Could you check a few things on this model? Use its own coordinates, in mm. A direction names the side the tool comes from. Coordinates: 2 decimals unless noted, no trailing zeros. Write each loop counter-clockwise with the first axis right and the second up, starting at its lowest first coordinate (ties: lowest second). Pieces come first, ordered by that corner, then holes. Notation, with made-up numbers: M 67.5,2 L 114.5,2 A10 ccw 114.5,6 Z; hole C 40.5,1 d8. An arc over 180 degrees is marked long. Answer as CSV lines item,"result". Start each with the question number.
Item 1: Suppose I cut it at A-A, the plane x = 7. Write out the boundary of the cut face in (y, z), and give its area (3 significant figures).
Item 2: We'd pull the mould along Z, two halves only. Please class faces 1 (the flat face through (0, 16, 0)), 2 (the cylindrical face through (2.854, -0.056, 42.939)), 3 (the cylindrical face through (11.19, -0.06, 62.72)), 4 (the flat face through (7, 4, 44)): +Z half, -Z half, draft (parallel to the pull), parting line (faces both ways), or undercut.
Item 3: I'm going to push flat-ended pins straight in: P1, Ø9.5, axis at x = -6, y = 43.5, coming from the +Z side; P2, Ø2.5, axis at x = 0.5, y = 0, coming from the -Z side; P3, Ø1.3, axis at x = 6.5, y = -12.5, coming from the +Z side. Where does each tip first touch, or does it pass through?
Item 4: Suppose I cut it at B-B, the plane y = 1. Write out the boundary of the cut face in (x, z), and give its area (3 significant figures).
Item 5: Suppose I cut it at D-D, the plane z = 4. Write out the boundary of the cut face in (x, y).
Item 6: Suppose I cut it at C-C, the plane y = -19. Write out the boundary of the cut face in (x, z), and give its area (3 significant figures).
Item 7: If I drill on line 1 along Z through (x, y) = (9, -13); line 2 along X through (y, z) = (-3, 7); line 3 along X through (y, z) = (-2.5, 52), over which ranges is the centre line in solid material (lowest first)? Write a range as [from, to].
Item 8: On a 3-axis mill with a long thin cutter (end or side, diameter ignored), from which of +Z, -Z, +X, -X, +Y, -Y can I reach the whole of each face in a straight line? I mean faces 5 (the flat face through (10.5, 39, 28)), 6 (the flat face through (-8, -12, 31.4)), 7 (the flat face through (13, 43, 22)). Say none if no direction works.
```python
from build123d import *

# Parameters (mm, degrees)
SKETCH4_W            = 31.4
SKETCH4_H            = 31.4
SKETCH4_W_2          = 25.4
SKETCH4_H_2          = 25.4
BOSS_EXTRUDE3_DEPTH  = 30
SKETCH5_W            = 31.4
SKETCH5_H            = 31.4
BOSS_EXTRUDE4_DEPTH  = 5
SKETCH6_W            = 31.4
SKETCH6_H            = 8
BOSS_EXTRUDE5_DEPTH  = 5
BOSS_EXTRUDE6_DEPTH  = 8
SKETCH8_R            = 9.5
BOSS_EXTRUDE7_DEPTH  = 8
SKETCH9_W            = 31.4
SKETCH9_H            = 10
BOSS_EXTRUDE8_DEPTH  = 5
SKETCH10_W           = 31.4
SKETCH10_H           = 10
BOSS_EXTRUDE9_DEPTH  = 11
SKETCH11_W           = 5.2
SKETCH11_H           = 10
BOSS_EXTRUDE10_DEPTH = 40
BOSS_EXTRUDE11_DEPTH = 3
SKETCH13_W           = 31.4
SKETCH13_H           = 31.4
CUT_EXTRUDE1_DEPTH   = 31.4
SKETCH15_W           = 31.4
SKETCH15_H           = 11
BOSS_EXTRUDE12_DEPTH = 12
SKETCH17_W           = 7.5
SKETCH17_H           = 31.4
BOSS_EXTRUDE13_DEPTH = 10
SKETCH18_R           = 3.75
BOSS_EXTRUDE14_DEPTH = 7.5
SKETCH19_W           = 3.6
SKETCH19_H           = 5
CUT_EXTRUDE2_DEPTH   = 31.4
CUT_EXTRUDE3_START   = 8
SKETCH8_2_R          = 9.5
CUT_EXTRUDE3_DEPTH   = 24
SKETCH20_W           = 9
SKETCH20_H           = 1
CUT_EXTRUDE4_DEPTH   = 26.4
SKETCH21_W           = 21
SKETCH21_H           = 13
CUT_EXTRUDE5_DEPTH   = 2


with BuildPart() as part:
    # Sketch4 → Boss-Extrude3 (new body)
    with BuildSketch(Plane.XY):
        Rectangle(SKETCH4_W, SKETCH4_H)
        Rectangle(SKETCH4_W_2, SKETCH4_H_2, mode=Mode.SUBTRACT)
    extrude(amount=BOSS_EXTRUDE3_DEPTH)

    # Sketch5 → Boss-Extrude4 (add)
    with BuildSketch(Plane.XY.offset(30)):
        Rectangle(SKETCH5_W, SKETCH5_H)
    extrude(amount=BOSS_EXTRUDE4_DEPTH)

    # Sketch6 → Boss-Extrude5 (add)
    with BuildSketch(Plane.XY.offset(35)):
        Rectangle(SKETCH6_W, SKETCH6_H)
    extrude(amount=BOSS_EXTRUDE5_DEPTH)

    # Sketch7 → Boss-Extrude6 (add)
    with BuildSketch(Plane.XZ.offset(4)):
        with BuildLine():
            Line((-15.7, 40), (-15.7, 52))
            ThreePointArc((-15.7, 52), (-11.306601718, 62.606601718), (-0.7, 67))
            Line((-0.7, 67), (0.7, 67))
            ThreePointArc((0.7, 67), (11.306601718, 62.606601718), (15.7, 52))
            Line((15.7, 52), (15.7, 40))
            Line((15.7, 40), (-15.7, 40))
        make_face()
    extrude(amount=-BOSS_EXTRUDE6_DEPTH)

    # Sketch8 → Boss-Extrude7 (add)
    with BuildSketch(Plane.XZ.offset(4)):
        with Locations(Location((0, 52, 0), (0, 0, 180))):
            Circle(SKETCH8_R)
    boss_extrude7 = extrude(amount=BOSS_EXTRUDE7_DEPTH)

    # Mirror1: Boss-Extrude7 across plane
    add(boss_extrude7.mirror(Plane.ZX))

    # Sketch9 → Boss-Extrude8 (add)
    with BuildSketch(Plane(origin=(0, 15.7, 0), x_dir=(1, 0, 0), z_dir=(0, 1, 0))):
        with Locations((0, -27)):
            Rectangle(SKETCH9_W, SKETCH9_H)
    extrude(amount=BOSS_EXTRUDE8_DEPTH)

    # Sketch10 → Boss-Extrude9 (add)
    with BuildSketch(Plane(origin=(0, 15.7, 0), x_dir=(1, 0, 0), z_dir=(0, 1, 0))):
        with Locations((0, -17)):
            Rectangle(SKETCH10_W, SKETCH10_H)
    extrude(amount=BOSS_EXTRUDE9_DEPTH)

    # Sketch11 → Boss-Extrude10 (add)
    with BuildSketch(Plane(origin=(0, 20.7, 0), x_dir=(1, 0, 0), z_dir=(0, 1, 0))):
        with Locations((-13.1, -27)):
            Rectangle(SKETCH11_W, SKETCH11_H)
        with Locations((13.1, -27)):
            Rectangle(SKETCH11_W, SKETCH11_H)
    extrude(amount=BOSS_EXTRUDE10_DEPTH)

    # Sketch12 → Boss-Extrude11 (add)
    with BuildSketch(Plane.XY.offset(32)):
        Polygon((-15.7, 60.7), (-10.5, 60.7), (-10.5, 20.7), (10.5, 20.7), (10.5, 60.7), (15.7, 60.7), (15.7, 15.7), (-15.7, 15.7), align=None)
    extrude(amount=BOSS_EXTRUDE11_DEPTH)

    # Sketch13 → Cut-Extrude1 (cut)
    with BuildSketch(Plane.ZY.offset(15.7)):
        with Locations((15.7, 0)):
            Rectangle(SKETCH13_W, SKETCH13_H)
    extrude(amount=-CUT_EXTRUDE1_DEPTH, mode=Mode.SUBTRACT)

    # Sketch15 → Boss-Extrude12 (add)
    with BuildSketch(Plane(origin=(0, 0, 12), x_dir=(-1, 0, 0), z_dir=(0, 0, -1))):
        with Locations((0, 21.2)):
            Rectangle(SKETCH15_W, SKETCH15_H)
    extrude(amount=BOSS_EXTRUDE12_DEPTH)

    # Sketch17 → Boss-Extrude13 (add)
    with BuildSketch(Plane.XZ.offset(-15.7)):
        with Locations((-8.25, 15.7)):
            Rectangle(SKETCH17_W, SKETCH17_H)
    boss_extrude13 = extrude(amount=BOSS_EXTRUDE13_DEPTH)

    # Sketch18 → Boss-Extrude14 (add)
    with BuildSketch(Plane.ZY.offset(12)):
        with BuildLine():
            Line((31.4, 5.7), (0, 5.7))
            Line((0, 5.7), (0, -13.3))
            ThreePointArc((0, -13.3), (4.393398282, -23.906601718), (15, -28.3))
            Line((15, -28.3), (16.4, -28.3))
            ThreePointArc((16.4, -28.3), (27.006601718, -23.906601718), (31.4, -13.3))
            Line((31.4, -13.3), (31.4, 5.7))
        make_face()
        with Locations((15.7, -13.3)):
            Circle(SKETCH18_R, mode=Mode.SUBTRACT)
    boss_extrude14 = extrude(amount=-BOSS_EXTRUDE14_DEPTH)

    # Mirror3: Boss-Extrude13, Boss-Extrude14 across plane
    add(boss_extrude13.mirror(Plane(origin=(0, 0, 0), x_dir=(0, 0, 1), z_dir=(1, 0, 0))))
    add(boss_extrude14.mirror(Plane(origin=(0, 0, 0), x_dir=(0, 0, 1), z_dir=(1, 0, 0))))

    # Sketch19 → Cut-Extrude2 (cut)
    with BuildSketch(Plane(origin=(15.7, 0, 0), x_dir=(0, 0, -1), z_dir=(1, 0, 0))):
        with Locations((-33.2, -13.2)):
            Rectangle(SKETCH19_W, SKETCH19_H)
    extrude(amount=-CUT_EXTRUDE2_DEPTH, mode=Mode.SUBTRACT)

    # Sketch8_2 → Cut-Extrude3 (cut)
    with BuildSketch(Plane.XZ.offset(4).offset(CUT_EXTRUDE3_START)):
        with Locations(Location((0, 52, 0), (0, 0, 270))):
            Circle(SKETCH8_2_R)
    extrude(amount=-CUT_EXTRUDE3_DEPTH, mode=Mode.SUBTRACT)

    # Sketch20 → Cut-Extrude4 (cut)
    with BuildSketch(Plane.XZ.offset(10.7)):
        with Locations((0, 31.9)):
            Rectangle(SKETCH20_W, SKETCH20_H)
    extrude(amount=-CUT_EXTRUDE4_DEPTH, mode=Mode.SUBTRACT)

    # Sketch21 → Cut-Extrude5 (cut)
    with BuildSketch(Plane(origin=(0, 20.7, 0), x_dir=(1, 0, 0), z_dir=(0, 1, 0))):
        with Locations((0, -28.5)):
            Rectangle(SKETCH21_W, SKETCH21_H)
    extrude(amount=-CUT_EXTRUDE5_DEPTH, mode=Mode.SUBTRACT)


solid = part.part
```
Ans:
1,outline,"M -28.3,15 A15 ccw -13.3,0 L 26.7,0 L 26.7,22 L 18.7,22 L 18.7,35 L 4,35 L 4,45.58 L -4,45.58 L -4,35 L -10.7,35 L -10.7,31.4 L -13.3,31.4 A15 ccw -28.3,16.4 Z; M -4,58.42 L 4,58.42 L 4,65.61 L -4,65.61 Z; hole C -13.3,15.7 d7.5"
1,area,"1,760 mm^2"
2,face 1,"-Z half"
2,face 2,"undercut"
2,face 3,"+Z half"
2,face 4,"draft"
3,P1,"stops at z = 35"
3,P2,"stops at z = 32.4"
3,P3,"stops at z = 31.4"
4,outline,"M -15.7,31.4 L -12,31.4 L -12,0 L -4.5,0 L -4.5,32.4 L 4.5,32.4 L 4.5,0 L 12,0 L 12,31.4 L 15.7,31.4 L 15.7,52 A15 ccw 0.7,67 L -0.7,67 A15 ccw -15.7,52 Z; hole C 0,52 d19"
4,area,"1,200 mm^2"
5,outline,"M -15.7,15.7 L -12,15.7 L -12,-23.5 L -4.5,-23.5 L -4.5,15.7 L 4.5,15.7 L 4.5,-23.5 L 12,-23.5 L 12,15.7 L 15.7,15.7 L 15.7,26.7 L -15.7,26.7 Z"
6,outline,"M -12,1.13 L -4.5,1.13 L -4.5,30.27 L -12,30.27 Z; M 4.5,1.13 L 12,1.13 L 12,30.27 L 4.5,30.27 Z"
6,area,"437 mm^2"
7,line 1,"z = [0, 11.96], [19.44, 31.4]"
7,line 2,"x = [-12, -4.5], [4.5, 12]"
7,line 3,"x = [-15.7, -9.5], [9.5, 15.7]"
8,face 5,"+Z, +Y"
8,face 6,"+Z, +X, -X, -Y"
8,face 7,"-Z, +X, -X, +Y"
